from build123d import *

# Parameters (mm, degrees)
SKETCH1_R             = 1.190050877
BOSS_EXTRUDE1_DEPTH   = 3.175
CUT_EXTRUDE1_DEPTH    = 4.175
SKETCH12_W            = 19.05
SKETCH12_H            = 23.8125
CUT_EXTRUDE2_DEPTH    = 4.175
SKETCH17_W            = 20.32
SKETCH17_H            = 20.32
CUT_EXTRUDE3_DEPTH    = 4.175
FILLET1_R             = 1.5875
F_6_CLEARANCE_HOLE1_D = 4.3053
CUT_EXTRUDE4_DEPTH    = 4.175
FILLET3_R             = 1.5875


with BuildPart() as part:
    # Sketch1 → Boss-Extrude1 (new body)
    with BuildSketch(Plane.XY):
        with BuildLine():
            Line((0, -17.78), (0, -141.2875))
            Line((0, -141.2875), (9.525, -141.2875))
            ThreePointArc((9.525, -141.2875), (30.833523511, -114.746148224), (45.72, -84.1375))
            Line((45.72, -84.1375), (45.72, -17.78))
            Line((45.72, -17.78), (0, -17.78))
        make_face()
        with Locations((18.7325, -40.894)):
            Circle(SKETCH1_R, mode=Mode.SUBTRACT)
    extrude(amount=-BOSS_EXTRUDE1_DEPTH)

    # Sketch11 → Cut-Extrude1 (cut, through all)
    with BuildSketch(Plane(origin=(20.844780046, -43.574770805, 0), x_dir=(1, 0, 0), z_dir=(0, 0, 1))):
        with BuildLine():
            Line((-5.443361979, 7.786170805), (1.218801886, 7.786170805))
            ThreePointArc((1.218801886, 7.786170805), (-2.112280046, -3.415229195), (-5.443361979, 7.786170805))
        make_face()
    extrude(amount=-CUT_EXTRUDE1_DEPTH, mode=Mode.SUBTRACT)

    # Sketch12 → Cut-Extrude2 (cut, through all)
    with BuildSketch(Plane.XY):
        with Locations((22.86, -68.54825)):
            Rectangle(SKETCH12_W, SKETCH12_H)
    extrude(amount=-CUT_EXTRUDE2_DEPTH, mode=Mode.SUBTRACT)

    # Sketch17 → Cut-Extrude3 (cut, through all)
    with BuildSketch(Plane.XY):
        with Locations((12.731722108, -106.422544949)):
            Rectangle(SKETCH17_W, SKETCH17_H)
    extrude(amount=-CUT_EXTRUDE3_DEPTH, mode=Mode.SUBTRACT)

    # Fillet1
    fillet1_edges = [part.edges().sort_by_distance(p)[0] for p in [
        (13.335, -80.4545, -1.5875),
        (13.335, -56.642, -1.5875),
        (32.385, -56.642, -1.5875),
        (32.385, -80.4545, -1.5875),
        (22.891722108, -96.262544949, -1.5875),
        (22.891722108, -116.582544949, -1.5875),
        (2.571722108, -116.582544949, -1.5875),
        (2.571722108, -96.262544949, -1.5875),
    ]]
    fillet(fillet1_edges, radius=FILLET1_R)

    # #6 Clearance Hole1 (through all)
    with Locations(Plane.XY):
        with Locations((9.144, -122.9995), (29.5275, -88.7095), (36.1315, -33.274)):
            Hole(F_6_CLEARANCE_HOLE1_D / 2)

    # Sketch20 → Cut-Extrude4 (cut, through all)
    with BuildSketch(Plane.XY):
        with BuildLine():
            Line((1.9875505, -93.544142926), (1.9875505, -82.303444681))
            ThreePointArc((1.9875505, -82.303444681), (2.002594465, -82.085411961), (2.04744123, -81.871511621))
            Line((2.04744123, -81.871511621), (3.907011168, -75.294806703))
            ThreePointArc((3.907011168, -75.294806703), (3.951857933, -75.080906363), (3.966901898, -74.862873644))
            Line((3.966901898, -74.862873644), (3.966901898, -59.18890883))
            ThreePointArc((3.966901898, -59.18890883), (4.431869883, -58.066376815), (5.554401898, -57.60140883))
            Line((5.554401898, -57.60140883), (9.117080567, -57.60140883))
            Line((9.117080567, -57.60140883), (27.511016487, -57.60140883))
            Line((27.511016487, -57.60140883), (27.511016487, -86.314118515))
            ThreePointArc((27.511016487, -86.314118515), (27.442924116, -86.774071456), (27.244488351, -87.194567028))
            ThreePointArc((27.244488351, -87.194567028), (26.786216014, -88.708422955), (27.244488351, -90.222278881))
            ThreePointArc((27.244488351, -90.222278881), (27.442924116, -90.642774454), (27.511016487, -91.102727395))
            Line((27.511016487, -91.102727395), (27.511016487, -93.544142926))
            ThreePointArc((27.511016487, -93.544142926), (27.046048502, -94.666674941), (25.923516487, -95.131642926))
            Line((25.923516487, -95.131642926), (3.5750505, -95.131642926))
            ThreePointArc((3.5750505, -95.131642926), (2.452518485, -94.666674941), (1.9875505, -93.544142926))
        make_face()
        with BuildLine():
            Line((39.239705373, -94.952090373), (41.119480948, -90.066805962))
            ThreePointArc((41.119480948, -90.066805962), (41.19867933, -89.78663398), (41.225378141, -89.49671003))
            Line((41.225378141, -89.49671003), (41.225378141, -81.903016886))
            ThreePointArc((41.225378141, -81.903016886), (40.760410156, -80.780484871), (39.637878141, -80.315516886))
            Line((39.637878141, -80.315516886), (36.61477648, -80.315516886))
            ThreePointArc((36.61477648, -80.315516886), (35.492244465, -80.780484871), (35.02727648, -81.903016886))
            Line((35.02727648, -81.903016886), (35.02727648, -87.180260326))
            ThreePointArc((35.02727648, -87.180260326), (34.917248136, -87.760978637), (34.602415054, -88.261198713))
            Line((34.602415054, -88.261198713), (33.520520126, -89.424866126))
            ThreePointArc((33.520520126, -89.424866126), (33.205687045, -89.925086202), (33.095658701, -90.505804513))
            Line((33.095658701, -90.505804513), (33.095658701, -94.381994441))
            ThreePointArc((33.095658701, -94.381994441), (33.560626686, -95.504526456), (34.683158701, -95.969494441))
            Line((34.683158701, -95.969494441), (37.758102566, -95.969494441))
            ThreePointArc((37.758102566, -95.969494441), (38.65674848, -95.690654737), (39.239705373, -94.952090373))
        make_face()
        with BuildLine():
            Line((20.217000424, -54.116093897), (14.306430977, -54.116093897))
            ThreePointArc((14.306430977, -54.116093897), (13.183898962, -53.651125912), (12.718930977, -52.528593897))
            Line((12.718930977, -52.528593897), (12.718930977, -50.013735278))
            ThreePointArc((12.718930977, -50.013735278), (13.183898962, -48.891203263), (14.306430977, -48.426235278))
            Line((14.306430977, -48.426235278), (20.217000424, -48.426235278))
            ThreePointArc((20.217000424, -48.426235278), (21.339532439, -48.891203263), (21.804500424, -50.013735278))
            Line((21.804500424, -50.013735278), (21.804500424, -52.528593897))
            ThreePointArc((21.804500424, -52.528593897), (21.339532439, -53.651125912), (20.217000424, -54.116093897))
        make_face()
        with BuildLine():
            Line((29.885101261, -44.237571754), (26.996152875, -44.237571754))
            ThreePointArc((26.996152875, -44.237571754), (25.87362086, -43.772603769), (25.408652875, -42.650071754))
            Line((25.408652875, -42.650071754), (25.408652875, -37.714249524))
            ThreePointArc((25.408652875, -37.714249524), (25.87362086, -36.591717509), (26.996152875, -36.126749524))
            Line((26.996152875, -36.126749524), (29.885101261, -36.126749524))
            ThreePointArc((29.885101261, -36.126749524), (31.007633276, -36.591717509), (31.472601261, -37.714249524))
            Line((31.472601261, -37.714249524), (31.472601261, -42.650071754))
            ThreePointArc((31.472601261, -42.650071754), (31.007633276, -43.772603769), (29.885101261, -44.237571754))
        make_face()
        with BuildLine():
            Line((20.406928746, -33.259078247), (14.243980141, -33.259078247))
            ThreePointArc((14.243980141, -33.259078247), (13.121448126, -32.794110262), (12.656480141, -31.671578247))
            Line((12.656480141, -31.671578247), (12.656480141, -28.136425111))
            ThreePointArc((12.656480141, -28.136425111), (13.121448126, -27.013893096), (14.243980141, -26.548925111))
            Line((14.243980141, -26.548925111), (20.406928746, -26.548925111))
            ThreePointArc((20.406928746, -26.548925111), (21.529460761, -27.013893096), (21.994428746, -28.136425111))
            Line((21.994428746, -28.136425111), (21.994428746, -31.671578247))
            ThreePointArc((21.994428746, -31.671578247), (21.529460761, -32.794110262), (20.406928746, -33.259078247))
        make_face()
        with BuildLine():
            Line((9.51166577, -50.881662937), (9.51166577, -29.220981566))
            ThreePointArc((9.51166577, -29.220981566), (9.046697786, -28.098449551), (7.92416577, -27.633481566))
            Line((7.92416577, -27.633481566), (4.736850702, -27.633481566))
            ThreePointArc((4.736850702, -27.633481566), (3.614318687, -28.098449551), (3.149350702, -29.220981566))
            Line((3.149350702, -29.220981566), (3.149350702, -50.881662937))
            ThreePointArc((3.149350702, -50.881662937), (3.614318687, -52.004194952), (4.736850702, -52.469162937))
            Line((4.736850702, -52.469162937), (7.92416577, -52.469162937))
            ThreePointArc((7.92416577, -52.469162937), (9.046697786, -52.004194952), (9.51166577, -50.881662937))
        make_face()
        with BuildLine():
            Line((40.313091041, -25.321573057), (4.684667753, -25.321573057))
            ThreePointArc((4.684667753, -25.321573057), (3.562135738, -24.856605072), (3.097167753, -23.734073057))
            Line((3.097167753, -23.734073057), (3.097167753, -20.606442704))
            ThreePointArc((3.097167753, -20.606442704), (3.562135738, -19.483910688), (4.684667753, -19.018942704))
            Line((4.684667753, -19.018942704), (40.313091041, -19.018942704))
            ThreePointArc((40.313091041, -19.018942704), (41.435623056, -19.483910688), (41.900591041, -20.606442704))
            Line((41.900591041, -20.606442704), (41.900591041, -23.734073057))
            ThreePointArc((41.900591041, -23.734073057), (41.435623056, -24.856605072), (40.313091041, -25.321573057))
        make_face()
        with BuildLine():
            Line((43.01404737, -76.302416551), (43.01404737, -60.74025149))
            ThreePointArc((43.01404737, -60.74025149), (42.549079385, -59.617719475), (41.42654737, -59.15275149))
            Line((41.42654737, -59.15275149), (35.637827713, -59.15275149))
            ThreePointArc((35.637827713, -59.15275149), (34.515295697, -59.617719475), (34.050327713, -60.74025149))
            Line((34.050327713, -60.74025149), (34.050327713, -76.302416551))
            ThreePointArc((34.050327713, -76.302416551), (34.515295697, -77.424948566), (35.637827713, -77.889916551))
            Line((35.637827713, -77.889916551), (41.42654737, -77.889916551))
            ThreePointArc((41.42654737, -77.889916551), (42.549079385, -77.424948566), (43.01404737, -76.302416551))
        make_face()
    extrude(amount=-CUT_EXTRUDE4_DEPTH, mode=Mode.SUBTRACT)

    # Fillet3
    fillet3_edges = [part.edges().sort_by_distance(p)[0] for p in [
        (13.464536443, -57.60140883, -1.5875),
        (27.511016487, -80.4545, -1.5875),
    ]]
    fillet(fillet3_edges, radius=FILLET3_R)


solid = part.part
The listing builds one solid part. Answer for the finished solid, in the listing's coordinates (mm). Give positions to 0.01 mm unless a question says otherwise; leave off trailing zeros. Order: outer loops, then holes, each group sorted by start corner. A loop starts at its lowest first (then second) coordinate and runs counter-clockwise, first axis right, second up. Notation, with made-up numbers: (-6.75, 46) - (32.25, 46) arc R17 cw to (32.25, 75) - close; hole circle Ø1 at (-3.75, 17). An arc over 180 degrees is marked (long way). Answer as CSV lines item,"result".
Q1. A cutting plane is placed at B-B, the plane x = 16.5. Determine the outline of the cut face in (y, z) (1 decimal).
Answer key:
outline,"(-133.9, -3.2) - (-116.6, -3.2) - (-116.6, 0) - (-133.9, 0) - close; (-96.3, -3.2) - (-95.1, -3.2) - (-95.1, 0) - (-96.3, 0) - close; (-56.6, -3.2) - (-54.1, -3.2) - (-54.1, 0) - (-56.6, 0) - close; (-48.4, -3.2) - (-46.6, -3.2) - (-46.6, 0) - (-48.4, 0) - close; (-35.8, -3.2) - (-33.3, -3.2) - (-33.3, 0) - (-35.8, 0) - close; (-26.5, -3.2) - (-25.3, -3.2) - (-25.3, 0) - (-26.5, 0) - close; (-19, -3.2) - (-17.8, -3.2) - (-17.8, 0) - (-19, 0) - close"
Q2. A cutting plane is placed at C-C, the plane z = -0.5. Count the separate pieces of the cut face and the enclosed holes in it, and give its area (3 significant figures).
Answer key:
separate pieces,"1"
enclosed holes,"13"
area,"2,350 mm^2"
Q3. Each of these flat-tipped pins is pushed along its axis until it touches: pin 1 Ø1 at (x, z) = (29.5, -1.5) entering from -Y; pin 2 Ø1.6 at (y, z) = (-86, -1) entering from +X; pin 3 Ø8 at (x, y) = (16.5, -112.5) entering from -Z. Where does it stop, or does it pass through?
Answer key:
pin 1,"stops at y = -117.57"
pin 2,"stops at x = 45.34"
pin 3,"passes through"
Q4. A cutting plane is placed at A-A, the plane y = -99.5. Determine the outline of the cut face in (x, z) (3 decimals).
Answer key:
outline,"(0, -3.175) - (2.572, -3.175) - (2.572, 0) - (0, 0) - close; (22.892, -3.175) - (39.308, -3.175) - (39.308, 0) - (22.892, 0) - close"
Q5. Straight lines are drawn through the part: L1, parallel to X at y = -31, z = -0.2; L2, parallel to X at y = -40.5, z = -0.3; L3, parallel to Y at x = 39, z = -1.8. For each, find the intervals that lie inside material, in ascending order.
Answer key:
L1,"x = 0 to 3.15, 9.51 to 12.66, 21.99 to 45.72"
L2,"x = 0 to 3.15, 9.51 to 12.65, 24.82 to 25.41, 31.47 to 45.72"
L3,"y = -100.13 to -95.37, -80.32 to -77.89, -59.15 to -25.32, -19.02 to -17.78"
Q6. Determine the mould class of faces 1 (the face through (33, -79, 0)), 2 (the face through (40.166, -92.544, -1.565)) for opening direction X: pulls with the +X half, pulls with the -X half, needs draft (parallel to the pull), parting line crosses it, or undercut.
Answer key:
face 1,"needs draft"
face 2,"undercut"
